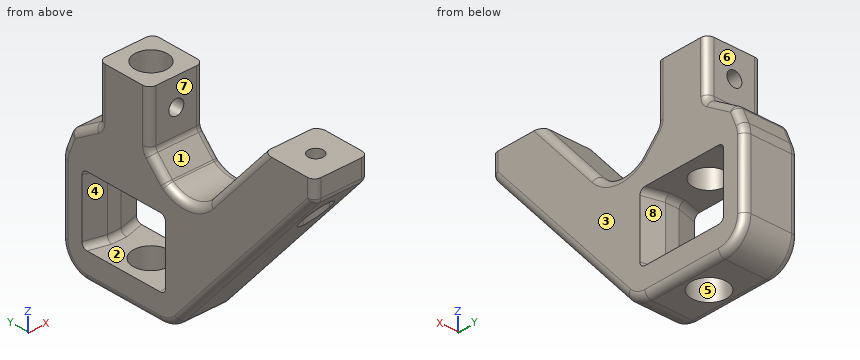
```python
from build123d import *
from OCP.BRepFilletAPI import BRepFilletAPI_MakeChamfer

# Parameters (mm, degrees)
SKETCH1_W                    = 25
SKETCH1_H                    = 29
BOSS_EXTRUDE1_DEPTH          = 10
SKETCH6_R                    = 5.9563
CUT_EXTRUDE1_DEPTH           = 113.716458426
CUT_EXTRUDE3_REACH           = 107.891
SKETCH14_R                   = 6.45
M5_START                     = -10
M5_CLEARANCE_HOLE1_OUTLINE_R = 2.75
M5_CLEARANCE_HOLE1_DEPTH     = 20
CUT_EXTRUDE2_DEPTH           = 18
M5_CLEARANCE_HOLE2_D         = 5.5
FILLET14_R                   = 12.7
FILLET13_R                   = 10
FILLET16_R                   = 2.54
CHAMFER1_SIZE                = 2
CHAMFER1_SIZE2               = 7.464101615
CHAMFER2_SIZE                = 2
CHAMFER2_SIZE2               = 7.464101615
FILLET17_R                   = 2


# Read off the part's stored shape, not the designer's step: M5 Clearance Hole1
with BuildPart() as part:
    # Sketch1 → Boss-Extrude1 (new, symmetric)
    with BuildSketch(Plane(origin=(0, 0, 0), x_dir=(0, 0, -1), z_dir=(1, 0, 0))):
        Polygon((7.460622198, -75), (72, -19.066312341), (72, 24.5), (35.01114111, 24.5), (27, 21.182154811), (20, 10), (0, 10), (0, -10), (20, -10), (27, -16.618919561), (40.474722748, -19.922182745), (0, -55), (0, -75), align=None)
        with Locations((49.5, 0)):
            Rectangle(SKETCH1_W, SKETCH1_H, mode=Mode.SUBTRACT)
    extrude(amount=BOSS_EXTRUDE1_DEPTH, both=True)

    # Sketch6 → Cut-Extrude1 (cut, through all)
    with BuildSketch(Plane(origin=(0, -81.5, -37), x_dir=(1, 0, 0), z_dir=(0, 0, 1))):
        with Locations(Location((0, 81.5, 0), (0, 0, 180))):
            Circle(SKETCH6_R)
    extrude(amount=CUT_EXTRUDE1_DEPTH, mode=Mode.SUBTRACT)

    # Sketch14 → Cut-Extrude3 (cut, up to next)
    with BuildSketch(Plane(origin=(0, -52.5, -72), x_dir=(1, 0, 0), z_dir=(0, 0, 1)), mode=Mode.PRIVATE) as cut_extrude3_sk1:
        with Locations(Location((0, 52.5, 0), (0, 0, 180))):
            Circle(SKETCH14_R)
    cut_extrude3_tool1 = extrude(cut_extrude3_sk1.sketch, amount=CUT_EXTRUDE3_REACH, mode=Mode.PRIVATE) & part.part
    add(cut_extrude3_tool1.solids().sort_by_distance((0, 0, -72))[0], mode=Mode.SUBTRACT)

    # M5 Clearance Hole1 outline → M5 Clearance Hole1 (cut)
    with BuildSketch(Plane(origin=(0, 0, 0), x_dir=(1, 0, 0), z_dir=(0, 1, 0)).offset(M5_START)):
        with Locations((0, 10)):
            Circle(M5_CLEARANCE_HOLE1_OUTLINE_R)
    extrude(amount=M5_CLEARANCE_HOLE1_DEPTH, mode=Mode.SUBTRACT)

    # Sketch10 → Cut-Extrude2 (cut)
    with BuildSketch(Plane.XY.offset(-30)):
        with BuildLine():
            ThreePointArc((5, -65), (3.535533906, -61.464466094), (0, -60))
            Line((0, -60), (0, -70))
            ThreePointArc((0, -70), (3.535533906, -68.535533906), (5, -65))
        make_face()
        with BuildLine():
            Line((0, -70), (0, -60))
            ThreePointArc((0, -60), (-5, -65), (0, -70))
        make_face()
    extrude(amount=CUT_EXTRUDE2_DEPTH, mode=Mode.SUBTRACT)

    # M5 Clearance Hole2 (through all)
    with Locations(Plane(origin=(0, 0, -12), x_dir=(-1, 0, 0), z_dir=(0, 0, -1))):
        with Locations((0, -65)):
            Hole(M5_CLEARANCE_HOLE2_D / 2)

    # Fillet14
    # the kernel refuses this fillet: 12.7 mm, written as the material it adds along each edge
    with BuildSketch(Plane(origin=(-10, -19.922182745, -40.474722748), x_dir=(0, 0.23809523809523664, 0.9712418121129117), z_dir=(1, 0, 0))) as fillet14_piece_1:
        with BuildLine():
            CenterArc((22.296336967, 9.505223671), FILLET14_R, 144.688307267, 83.767361366)
            Line((11.932887465, 16.846130592), (11.725618475, 16.992948731))
            Line((11.725618475, 16.992948731), (-0.20726899, 0.146818138))
            Line((-0.20726899, 0.146818138), (0, -0.254))
            ThreePointArc((0, -0.254), (6.936852687, -0.254), (13.705252742, -0.190104473))
            Line((13.705252742, -0.190104473), (13.873705374, 0))
        make_face()
    extrude(amount=20)

    # Fillet13
    fillet13_edges = [part.edges().sort_by_distance(p)[0] for p in [
        (0, 24.5, -35.01114111),
        (0, 24.5, -72),
        (0, -19.066312341, -72),
    ]]
    fillet(fillet13_edges, radius=FILLET13_R)

    # Fillet16
    fillet16_edges = [part.edges().sort_by_distance(p)[0] for p in [
        (10, -48.528458156, -38.004949088),
        (10, 0, -72),
        (10, -18.653747718, -71.096503718),
        (10, 21.571067812, -69.071067812),
        (10, 24.307902492, -35.049346594),
        (-10, 10, -10),
        (-10, 15.591077405, -23.5),
        (-10, -75, -3.730311099),
        (-10, -13.30945978, -23.5),
        (-10, -10, -10),
        (10, -10, -10),
        (10, -13.30945978, -23.5),
        (0, 10, -20),
        (0, 21.182154811, -27),
        (0, -75, -7.460622198),
        (0, -16.618919561, -27),
        (0, -10, -20),
        (10, -75, -3.730311099),
        (10, 15.591077405, -23.5),
        (10, 10, -10),
        (-10, -44.221342733, -12.437010014),
        (10, -44.221342733, -12.437010014),
        (-10, -25.437608609, -29.156236253),
        (10, -25.437608609, -29.156236253),
        (-10, 22.460572534, -30.08681816),
        (10, 22.460572534, -30.08681816),
        (-10, 24.5, -49.5),
        (-10, 0, -72),
        (-10, -48.528458156, -38.004949088),
        (-10, -18.653747718, -71.096503718),
        (-10, 21.571067812, -69.071067812),
        (-10, 24.307902492, -35.049346594),
        (10, 24.5, -49.5),
    ]]
    fillet(fillet16_edges, radius=FILLET16_R)

    # Chamfer1: one chamfer whose edges measure the first distance from different faces: ONE call of the kernel's chamfer builder (chamfer() names one face for all edges)
    chamfer1_edges_1 = [part.edges().sort_by_distance(p)[0] for p in [
        (10, 14.5, -49.5),
    ]]
    chamfer1_side_1 = [part.faces().sort_by_distance(p)[0] for p in [
        (10, -18.267082867, -33.779126771),
    ]]
    chamfer1_edges_2 = [part.edges().sort_by_distance(p)[0] for p in [
        (-10, 14.5, -49.5),
    ]]
    chamfer1_side_2 = [part.faces().sort_by_distance(p)[0] for p in [
        (-10, -18.267082867, -33.779126771),
    ]]
    chamfer1 = BRepFilletAPI_MakeChamfer(part.part.solid().wrapped)
    for e in chamfer1_edges_1:
        chamfer1.Add(CHAMFER1_SIZE, CHAMFER1_SIZE2, e.wrapped, chamfer1_side_1[0].wrapped)  # the first distance lies on this face
    for e in chamfer1_edges_2:
        chamfer1.Add(CHAMFER1_SIZE, CHAMFER1_SIZE2, e.wrapped, chamfer1_side_2[0].wrapped)  # the first distance lies on this face
    add(Compound.cast(chamfer1.Shape()), mode=Mode.REPLACE)

    # Chamfer2: one chamfer whose edges measure the first distance from different faces: ONE call of the kernel's chamfer builder (chamfer() names one face for all edges)
    chamfer2_edges_1 = [part.edges().sort_by_distance(p)[0] for p in [
        (-10, -14.5, -49.5),
    ]]
    chamfer2_side_1 = [part.faces().sort_by_distance(p)[0] for p in [
        (-10, -18.927449514, -33.471681192),
    ]]
    chamfer2_edges_2 = [part.edges().sort_by_distance(p)[0] for p in [
        (10, -14.5, -49.5),
    ]]
    chamfer2_side_2 = [part.faces().sort_by_distance(p)[0] for p in [
        (10, -18.927449514, -33.471681192),
    ]]
    chamfer2 = BRepFilletAPI_MakeChamfer(part.part.solid().wrapped)
    for e in chamfer2_edges_1:
        chamfer2.Add(CHAMFER2_SIZE, CHAMFER2_SIZE2, e.wrapped, chamfer2_side_1[0].wrapped)  # the first distance lies on this face
    for e in chamfer2_edges_2:
        chamfer2.Add(CHAMFER2_SIZE, CHAMFER2_SIZE2, e.wrapped, chamfer2_side_2[0].wrapped)  # the first distance lies on this face
    add(Compound.cast(chamfer2.Shape()), mode=Mode.REPLACE)

    # Fillet17
    fillet17_edges = [part.edges().sort_by_distance(p)[0] for p in [
        (0, 14.5, -62),
        (0, 14.5, -37),
        (6.267949192, 15.5, -37),
        (6.267949192, 15.5, -62),
        (-6.267949192, 15.5, -37),
        (-6.267949192, 15.5, -62),
        (0, -14.5, -37),
        (0, -14.5, -62),
        (-6.267949192, -15.5, -62),
        (-6.267949192, -15.5, -37),
        (6.267949192, -15.5, -62),
        (6.267949192, -15.5, -37),
    ]]
    fillet(fillet17_edges, radius=FILLET17_R)


solid = part.part
```
The listing builds one solid part. Answer for the finished solid, in the listing's coordinates (mm). Face numbers are marked on the shaded views. A direction names the side the tool comes from. Give positions to 0.01 mm unless a question says otherwise; leave off trailing zeros. Order: outer loops, then holes, each group sorted by start corner. A loop starts at its lowest first (then second) coordinate and runs counter-clockwise, first axis right, second up. Notation, with made-up numbers: (36, 70.5) -> (58, 70.5) arc R11 cw to (58, 84.5) -> close; hole circle Ø11 at (36.25, -11). An arc over 180 degrees is marked (long way). Answer as CSV lines item,"result". Start each with the question number.
Q1. Which of the six approach directions +Z, -Z, +X, -X, +Y, -Y give full straight-line access (tool end or side, diameter ignored) to the marked faces 4, 5, 6, 7 and 8?
Q2. Find the intervals of material crossed by L1, parallel to Y at x = 5, z = -22; L2, parallel to X at y = -6.5, z = -9; L3, parallel to X at y = -7.55, z = -10, in increasing order.
Q3. Determine the mould class of the marked faces 1, 2 and 3 for opening direction Z: pulls with the +Z half, pulls with the -Z half, needs draft (parallel to the pull), parting line crosses it, or undercut.
Q4. A cutting plane is placed at A-A (y = 0). Determine the outline of the cut face in (x, z).
Q5. Given pin 1 (10 mm diameter, centred on x = -5, y = -50.5, fed in from +Z); pin 2 (6.5 mm diameter, centred on x = 0, z = -10, fed in from +Y); pin 3 (6 mm diameter, centred on x = 3, y = -45, fed in from +Z); pin 4 (2.5 mm diameter, centred on x = 0.5, z = -49, fed in from -Y), each flat-ended and moving along its own axis, determine where each tip first touches the part or whether it passes through.
Results found:
1,face 4,"-X"
1,face 5,"-Z"
1,face 6,"+Z, +X, -X, +Y"
1,face 7,"+Z, +X, -X"
1,face 8,"+X"
2,L1,"-62.4 to -35.93, -11.89 to -3.24, 3.24 to 13.19"
2,L2,"-10 to -2.56, 2.56 to 10"
2,L3,"-10 to -2.75, 2.75 to 10"
3,face 1,"pulls with the +Z half"
3,face 2,"undercut"
3,face 3,"needs draft"
4,outline,"(-10, -69.46) arc R2.54 ccw to (-7.46, -72) -> (-6.45, -72) -> (-6.45, -62) -> (-10, -62) -> close; (-10, -37) -> (-5.96, -37) -> (-5.96, 0) -> (-10, 0) -> close; (5.96, -37) -> (10, -37) -> (10, 0) -> (5.96, 0) -> close; (6.45, -72) -> (7.46, -72) arc R2.54 ccw to (10, -69.46) -> (10, -62) -> (6.45, -62) -> close"
5,pin 1,"z = 0"
5,pin 2,"y = 10"
5,pin 3,"z = -8.08"
5,pin 4,"y = -40.08"
